```python
from build123d import *
from build123d.topology import SkipClean

# Parameters (mm, degrees)
SKETCH1_R                   = 6.35
FLANGE_BOTTOM_DEPTH         = 7.9248
SKETCH2_R                   = 6.35
FLANGMIDBODY_DEPTH          = 3.175
FLANGELEGS_DEPTH            = 11.1252
FILLET1_R                   = 3.175
LOCKINGSHAFTHOLE_DEPTH      = 22.060567449
LOCKINGSHAFTHOLE_DEPTH_BACK = 22.060567449
SKETCH4_R                   = 1.27
FILLET3_R                   = 1.27
SKETCH5_R                   = 3.17246
CENTERSHAFTHOLE_DEPTH       = 24.97072446
SKETCH11_R                  = 0.873550069
SET_SCREW_DEPTH             = 22.060567459
SKETCH12_R                  = 0.873550069
SUB_DRILL_DEPTH             = 1.27


# Some blends are built 0.0001 mm under size
with BuildPart() as part:
    # Sketch1 → Flange Bottom (new body)
    with BuildSketch(Plane(origin=(-19.05, 0, 0), x_dir=(0, 0, -1), z_dir=(1, 0, 0))):
        Circle(SKETCH1_R)
    extrude(amount=FLANGE_BOTTOM_DEPTH)

    # Sketch2 → Flangmidbody (add)
    with BuildSketch(Plane(origin=(-11.1252, 0, 0), x_dir=(0, 0, -1), z_dir=(1, 0, 0))):
        Circle(SKETCH2_R)
    extrude(amount=FLANGMIDBODY_DEPTH)

    # Sketch3 → Flangelegs (add)
    with SkipClean():  # the faces are left unmerged after this step: merging them gives an invalid solid
        with BuildSketch(Plane(origin=(-7.9502, 0, 0), x_dir=(0, 0, -1), z_dir=(1, 0, 0))):
            with BuildLine():
                Line((-5.499261314, 3.175), (-3.965573729, 3.175))
                ThreePointArc((-3.965573729, 3.175), (-5.08, 0), (-3.965573729, -3.175))
                Line((-3.965573729, -3.175), (-5.499261314, -3.175))
                ThreePointArc((-5.499261314, -3.175), (-6.35, 0), (-5.499261314, 3.175))
            make_face()
            with BuildLine():
                Line((3.965573729, 3.175), (5.499261314, 3.175))
                ThreePointArc((5.499261314, 3.175), (6.35, 0), (5.499261314, -3.175))
                Line((5.499261314, -3.175), (3.965573729, -3.175))
                ThreePointArc((3.965573729, -3.175), (5.08, 0), (3.965573729, 3.175))
            make_face()
        extrude(amount=FLANGELEGS_DEPTH)

    # Fillet1
    fillet1_edges = [part.edges().sort_by_distance(p)[0] for p in [
        (3.175, -3.175, -4.732417522),
        (3.175, 3.175, -4.732417522),
        (3.175, -3.175, 4.732417522),
        (3.175, 3.175, 4.732417522),
    ]]
    fillet(fillet1_edges, radius=FILLET1_R - 0.0001)  # a hair under: the kernel refuses the full size

    # Sketch4 → Lockingshafthole (cut, two sides: drawn at the far end of the back side and taken through both)
    with BuildSketch(Plane.XY.offset(-LOCKINGSHAFTHOLE_DEPTH_BACK)):
        Circle(SKETCH4_R)
    extrude(amount=LOCKINGSHAFTHOLE_DEPTH + LOCKINGSHAFTHOLE_DEPTH_BACK, mode=Mode.SUBTRACT)

    # Fillet3
    # the kernel refuses this fillet: 1.27 mm, written as the material it adds along each edge
    with BuildSketch(Plane(origin=(-7.9502, 3.175, -0.790573729), x_dir=(1, 0, 0), z_dir=(0, 0, -1))) as fillet3_piece_1_section:
        with BuildLine():
            CenterArc((FILLET3_R, -FILLET3_R), FILLET3_R, 90, 90)
            Line((0, -FILLET3_R), (0, 0))
            Line((0, 0), (FILLET3_R, 0))
        make_face()
    fillet3_piece_1 = extrude(amount=7.883687585, mode=Mode.PRIVATE)
    fillet3_piece_1 = fillet3_piece_1 & Plane(origin=(-7.671308244, 0, 0), x_dir=(0, 0.4999999999999997, -0.8660254037844388), z_dir=(-1, 0, 0)) * Cylinder(6.35, 21, mode=Mode.PRIVATE)
    fillet3_piece_1 = fillet3_piece_1 - Plane(origin=(-7.671308244, 0, 0), x_dir=(0, -0.6249999999999998, -0.7806247497997999), z_dir=(-1, 0, 0)) * Cylinder(5.08, 21, mode=Mode.PRIVATE)
    add(fillet3_piece_1)
    with BuildSketch(Plane(origin=(-7.9502, -3.175, -8.674261314), x_dir=(1, 0, 0), z_dir=(0, 0, 1))) as fillet3_piece_2_section:
        with BuildLine():
            CenterArc((FILLET3_R, -FILLET3_R), FILLET3_R, 90, 90)
            Line((0, -FILLET3_R), (0, 0))
            Line((0, 0), (FILLET3_R, 0))
        make_face()
    fillet3_piece_2 = extrude(amount=7.883687585, mode=Mode.PRIVATE)
    fillet3_piece_2 = fillet3_piece_2 & Plane(origin=(-7.671308757, 0, 0), x_dir=(0, 0.4999999999999997, -0.8660254037844388), z_dir=(-1, 0, 0)) * Cylinder(6.35, 21, mode=Mode.PRIVATE)
    fillet3_piece_2 = fillet3_piece_2 - Plane(origin=(-7.671308757, 0, 0), x_dir=(0, -0.6249999999999998, -0.7806247497997999), z_dir=(-1, 0, 0)) * Cylinder(5.08, 21, mode=Mode.PRIVATE)
    add(fillet3_piece_2)
    with BuildSketch(Plane(origin=(-7.9502, -3.175, 0.790573729), x_dir=(0, -1, 0), z_dir=(0, 0, 1))) as fillet3_piece_3_section:
        with BuildLine():
            CenterArc((FILLET3_R, FILLET3_R), FILLET3_R, 180, 90)
            Line((0, FILLET3_R), (0, 0))
            Line((0, 0), (FILLET3_R, 0))
        make_face()
    fillet3_piece_3 = extrude(amount=7.883687585, mode=Mode.PRIVATE)
    fillet3_piece_3 = fillet3_piece_3 & Plane(origin=(-7.671308363, 0, 0), x_dir=(0, 0, -1), z_dir=(-1, 0, 0)) * Cylinder(6.35, 21, mode=Mode.PRIVATE)
    fillet3_piece_3 = fillet3_piece_3 - Plane(origin=(-7.671308363, 0, 0), x_dir=(0, 0.6250000000000004, 0.7806247497997995), z_dir=(-1, 0, 0)) * Cylinder(5.08, 21, mode=Mode.PRIVATE)
    add(fillet3_piece_3)
    with BuildSketch(Plane(origin=(-7.9502, 3.175, 8.674261314), x_dir=(0, 1, 0), z_dir=(0, 0, -1))) as fillet3_piece_4_section:
        with BuildLine():
            CenterArc((FILLET3_R, FILLET3_R), FILLET3_R, 180, 90)
            Line((0, FILLET3_R), (0, 0))
            Line((0, 0), (FILLET3_R, 0))
        make_face()
    fillet3_piece_4 = extrude(amount=7.883687585, mode=Mode.PRIVATE)
    fillet3_piece_4 = fillet3_piece_4 & Plane(origin=(-7.671308731, 0, 0), x_dir=(0, 0, -1), z_dir=(-1, 0, 0)) * Cylinder(6.35, 21, mode=Mode.PRIVATE)
    fillet3_piece_4 = fillet3_piece_4 - Plane(origin=(-7.671308731, 0, 0), x_dir=(0, 0.6250000000000004, 0.7806247497997995), z_dir=(-1, 0, 0)) * Cylinder(5.08, 21, mode=Mode.PRIVATE)
    add(fillet3_piece_4)

    # Sketch5 → CenterShaftHole (cut, through all)
    with BuildSketch(Plane.ZY.offset(19.05)):
        Circle(SKETCH5_R)
    extrude(amount=-CENTERSHAFTHOLE_DEPTH, mode=Mode.SUBTRACT)

    # Sketch11 → Set Screw (cut, through all)
    with BuildSketch(Plane(origin=(0, 0, 0), x_dir=(1, 0, 0), z_dir=(0, 1, 0))):
        with Locations(Location((-15.0876, 0, 0), (0, 0, 270))):
            Circle(SKETCH11_R)
    extrude(amount=-SET_SCREW_DEPTH, mode=Mode.SUBTRACT)

    # Sketch12 → Sub Drill (cut)
    with BuildSketch(Plane.XY.offset(-6.35)):
        with Locations((-15.0876, 0)):
            Circle(SKETCH12_R)
    extrude(amount=SUB_DRILL_DEPTH, mode=Mode.SUBTRACT)


solid = part.part
```
Geometry check sheet. Reference: the model listing, model coordinates, mm. A direction names the side the tool comes from. Coordinates: 2 decimals unless noted, no trailing zeros. Order: outer loops, then holes, each group sorted by start corner. A loop starts at its lowest first (then second) coordinate and runs counter-clockwise, first axis right, second up. Notation, with made-up numbers: M 86.25,38.5 L 110.25,38.5 A17 ccw 110.25,68.5 Z; hole C 77,3.25 d10. An arc over 180 degrees is marked long. Answer as a JSON object with one key per item and string values.
Q1. Tool access check on faces 5 (the cylindrical face through (-10.563, 5.876, -2.406)), 6 (the cylindrical face through (-14.254, 0.262, -5.724)), 7 (the flat face through (-3, -3.175, -5)), 8 (the flat face through (-7.95, 0.1, 3.5)), 9 (the flat face through (-3, 3.175, -5)). Record the directions out of +Z, -Z, +X, -X, +Y, -Y that give a thin tool (end or side, any length) a straight path to the whole face; none if there is none.
Results are:
{"face 5": "+X, -X", "face 6": "-Z", "face 7": "+Z, -Z, +X, -Y", "face 8": "+X", "face 9": "+Z, -Z, +X, +Y"}
Q2. Scan lines: line 1 (X direction, y = 0, z = -5.65) (3 decimals); line 2 (X direction, y = 0, z = 6.05) (3 decimals); line 3 (Y direction, x = -14, z = 0). Record each from-to range of solid material in increasing order.
Results are:
{"line 1": "x = -19.05 to -15.961, -14.214 to -1.27, 1.27 to 3.175", "line 2": "x = -19.05 to -1.27, 1.27 to 3.175", "line 3": "y = -6.35 to -3.17, 3.17 to 6.35"}
Q3. Release check for a two-part mould opening along Z. For faces 1 (the cylindrical face through (-15.94, -4.68, -0.19)), 2 (the cylindrical face through (-13.578, 3.145, -0.413)), 3 (the flat face through (-15, 0, -5.08)), 4 (the flat face through (-3, -3.175, 5)) record: released by +Z, released by -Z, zero draft, split by the parting line, or undercut.
Results are:
{"face 1": "undercut", "face 2": "undercut", "face 3": "released by -Z", "face 4": "zero draft"}
Q4. Cross-section at A-A on z = 0. Record the cut outline in (x, y), and give its area (3 significant figures).
Results are:
{"outline": "M -19.05,-6.35 L -15.96,-6.35 L -15.96,-3.17 L -19.05,-3.17 Z; M -19.05,3.17 L -7.95,3.17 L -7.95,6.35 L -19.05,6.35 Z; M -14.21,-6.35 L -7.95,-6.35 L -7.95,-3.17 L -14.21,-3.17 Z", "area": "65.0 mm²"}
Q5. Depth check by flat-ended pin: pin 1 Ø1.5 at (x, z) = (-15.5, 4.5) entering from -Y; pin 2 Ø0.5 at (x, z) = (-2, 4.5) entering from -Y (3 decimals); pin 3 Ø1.7 at (x, z) = (-2, 5) entering from +Y (3 decimals); pin 4 Ø5.5 at (y, z) = (0, 0) entering from -X. Enter the tip coordinate at first touch or a pass-through.
Results are:
{"pin 1": "stops at y = -5.12", "pin 2": "stops at y = -3.175", "pin 3": "stops at y = 3.175", "pin 4": "passes through"}
Q6. Cross-section at B-B on x = -4. Record the cut outline in (y, z) (3 decimals), and give its area (3 significant figures).
Results are:
{"outline": "M -3.175,-5.499 A6.35 ccw 3.175,-5.499 L 3.175,-3.966 A5.08 cw -3.175,-3.966 Z; M -3.175,3.966 A5.08 cw 3.175,3.966 L 3.175,5.499 A6.35 ccw -3.175,5.499 Z", "area": "17.1 mm²"}
Q7. Cross-section at C-C on x = 1. Record the cut outline in (y, z).
Results are:
{"outline": "M -3.01,-5.59 A6.35 ccw -0.78,-6.3 L -0.78,-5.02 A5.08 cw -3.01,-4.09 Z; M -3.01,4.09 A5.08 cw -0.78,5.02 L -0.78,6.3 A6.35 ccw -3.01,5.59 Z; M 0.78,-6.3 A6.35 ccw 3.01,-5.59 L 3.01,-4.09 A5.08 cw 0.78,-5.02 Z; M 0.78,5.02 A5.08 cw 3.01,4.09 L 3.01,5.59 A6.35 ccw 0.78,6.3 Z"}
